Answer from the drawing. Dimensions are ordinates in mm from the lowest x, y and z of the part. A direction names the side the tool comes from. Coordinates: 2 decimals unless noted, no trailing zeros. Write each loop counter-clockwise with the first axis right and the second up, starting at its lowest first coordinate (ties: lowest second). Pieces come first, ordered by that corner, then holes.
(1) Which of the six approach directions +Z, -Z, +X, -X, +Y, -Y give full straight-line access (tool end or side, diameter ignored) to the marked faces 1, 2, 3, 4 and 5?
(2) Given pin 1 (6.5 mm diameter, centred on x = 0.36, y = 12, fed in from -Z); pin 2 (12 mm diameter, centred on y = 22, z = 15, fed in from -X) (1 decimal); pin 3 (0.5 mm diameter, centred on x = 29.5, z = 18.5, fed in from +Y), each flat-ended and moving along its own axis, determine where each tip first touches the part or whether it passes through.
(3) Find the intervals of material crossed by probe 1 along Z at (x, y) = (18.5, 6); probe 2 along X at (y, z) = (22.75, 12.25); probe 3 along X at (y, z) = (12, 18.6), in increasing order.
(4) Section A-A on y = 12 is taken. Write down the section's boundary in (x, z).
(5) Section B-B on z = 4 is taken. Write down the section's boundary in (x, y).
(6) Section D-D on y = 5.5 is taken. Write down the section's boundary in (x, z), then the cut area to 3 significant figures.
(7) Section C-C on x = 24 is taken. Write down the section's boundary in (y, z).
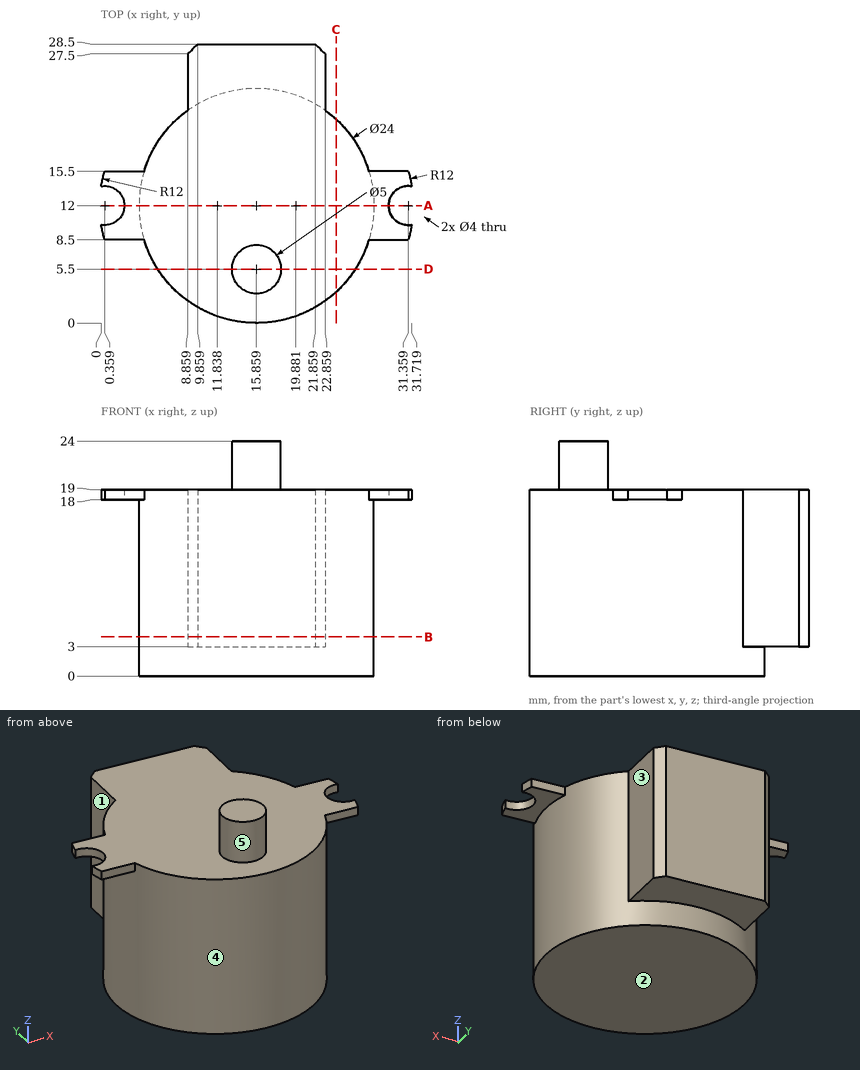
Response:
1. face 1: +Z, -Z, -X, +Y
1. face 2: -Z, +X, -X, +Y, -Y
1. face 3: +Z, -Z, +X, +Y
1. face 4: -Z
1. face 5: +Z
2. pin 1: stops at z = 18
2. pin 2: stops at x = 4.5
2. pin 3: stops at y = 15.5
3. probe 1: z = 0 to 19
3. probe 2: x = 8.86 to 22.86
3. probe 3: x = 2.36 to 29.36
4. outline: (2.36, 18) - (3.86, 18) - (3.86, 0) - (27.86, 0) - (27.86, 18) - (29.36, 18) - (29.36, 19) - (2.36, 19) - close
5. outline: (8.86, 21.75) arc R12 ccw (long way) to (22.86, 21.75) - (22.86, 27.5) - (21.86, 28.5) - (9.86, 28.5) - (8.86, 27.5) - close
6. outline: (5.77, 0) - (25.95, 0) - (25.95, 19) - (18.36, 19) - (18.36, 24) - (13.36, 24) - (13.36, 19) - (5.77, 19) - close
6. area: 408 mm2
7. outline: (3.18, 0) - (20.82, 0) - (20.82, 19) - (3.18, 19) - close
